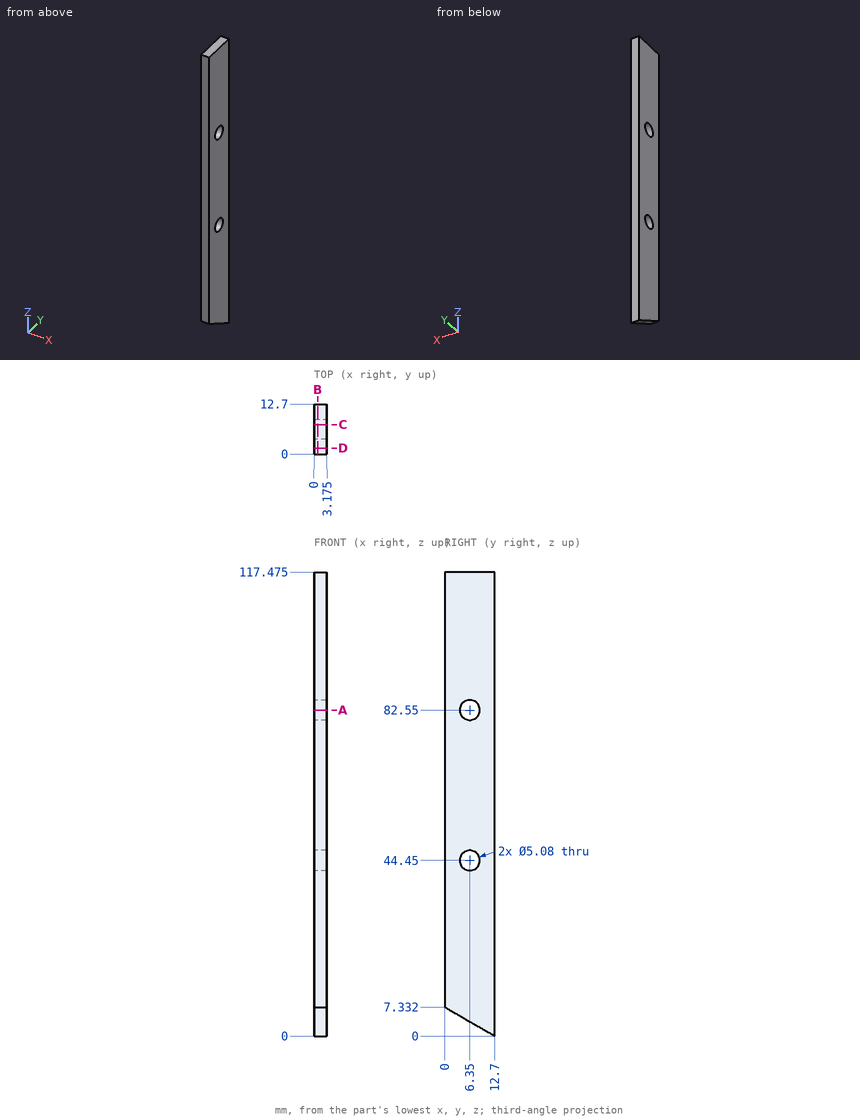
Answer from the drawing. Dimensions are ordinates in mm from the lowest x, y and z of the part. Give positions to 0.01 mm unless a question says otherwise; leave off trailing zeros. Order: outer loops, then holes, each group sorted by start corner. A loop starts at its lowest first (then second) coordinate and runs counter-clockwise, first axis right, second up.
(1) Find section B-B (x = 0.9). Give the number of separate pieces and of enclosed holes in the cut face, plus the area to 4 significant figures.
(2) Straight lines are drawn through the part: L1, parallel to Z at x = 2.1, y = 5 (1 decimal); L2, parallel to Z at x = 2.15, y = 6.35 (1 decimal); L3, parallel to Y at x = 0.5, z = 81. For each, find the intervals that lie inside material, in ascending order.
(3) Find section D-D (y = 1.5). Give the vertices of the cut face in (x, z) (1 decimal).
(4) Find section C-C (y = 7.5). Give the vertices of the cut face in (x, z) (1 decimal).
(5) Given pin 1 (6 mm diameter, centred on y = 6.35, z = 82.55, fed in from -X); pin 2 (3 mm diameter, centred on y = 6.35, z = 44.45, fed in from -X), each flat-ended and moving along its own axis, determine where each tip first touches the part or whether it passes through.
(6) Find section A-A (z = 82.55). Give the vertices of the cut face in (x, y) (1 decimal).
Result sheet:
1. separate pieces: 1
1. enclosed holes: 2
1. area: 1,405 mm2
2. L1: z = 4.4 to 42.3, 46.6 to 80.4, 84.7 to 117.5
2. L2: z = 3.7 to 41.9, 47 to 80, 85.1 to 117.5
2. L3: y = 0 to 4.34, 8.36 to 12.7
3. outline: (0, 6.5) - (3.2, 6.5) - (3.2, 117.5) - (0, 117.5) - close
4. outline: (0, 3) - (3.2, 3) - (3.2, 42.2) - (0, 42.2) - close; (0, 46.7) - (3.2, 46.7) - (3.2, 80.3) - (0, 80.3) - close; (0, 84.8) - (3.2, 84.8) - (3.2, 117.5) - (0, 117.5) - close
5. pin 1: stops at x = 0
5. pin 2: passes through
6. outline: (0, 0) - (3.2, 0) - (3.2, 3.8) - (0, 3.8) - close; (0, 8.9) - (3.2, 8.9) - (3.2, 12.7) - (0, 12.7) - close
